Source: CAD feature listing. Evaluate the final solid. Frame: model axes, mm. Coordinates: 2 decimals unless noted, no trailing zeros. Write each loop counter-clockwise with the first axis right and the second up, starting at its lowest first coordinate (ties: lowest second). Pieces come first, ordered by that corner, then holes. Notation, with made-up numbers: (-7, 13) - (8, 13) arc R11 cw to (8, 17) - close; hole circle Ø10 at (44, 81.25). An arc over 180 degrees is marked (long way). One line per item, written item: value.
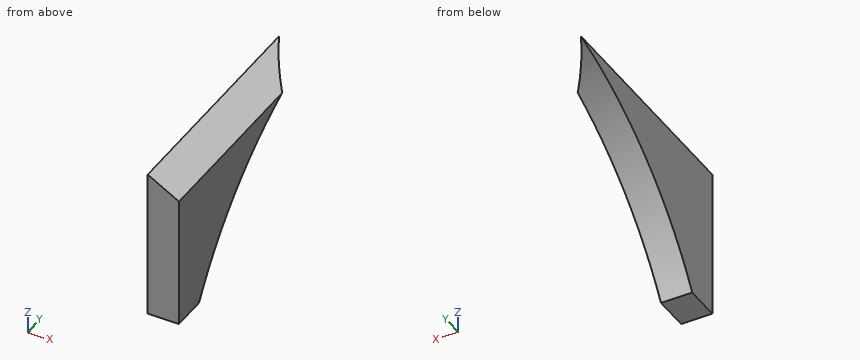
from build123d import *

# Parameters (mm, degrees)
BOSS_EXTRUDE1_DEPTH = 4
SKETCH2_W           = 10.75
SKETCH2_H           = 20.327264221
CUT_EXTRUDE1_DEPTH  = 4
CUT_EXTRUDE2_DEPTH  = 50.8


with BuildPart() as part:
    # Sketch1 → Boss-Extrude1 (new body)
    with BuildSketch(Plane(origin=(0, 0, 0), x_dir=(0, 0, -1), z_dir=(1, 0, 0))):
        with BuildLine():
            Line((-11.867139326, 22.331980986), (-11.867139326, -7.668019014))
            Line((-11.867139326, -7.668019014), (18.132860674, -7.668019014))
            ThreePointArc((18.132860674, -7.668019014), (-0.870157122, 3.328963189), (-11.867139326, 22.331980986))
        make_face()
    extrude(amount=BOSS_EXTRUDE1_DEPTH)

    # Sketch2 → Cut-Extrude1 (cut)
    with BuildSketch(Plane(origin=(4, 0, 0), x_dir=(0, 0, -1), z_dir=(1, 0, 0))):
        with Locations((12.757860674, 2.495613097)):
            Rectangle(SKETCH2_W, SKETCH2_H)
    extrude(amount=-CUT_EXTRUDE1_DEPTH, mode=Mode.SUBTRACT)

    # Sketch3 → Cut-Extrude2 (cut)
    with BuildSketch(Plane.XZ.offset(7.668019014)):
        Polygon((0, 11.867139326), (4, 9.557738249), (4, 11.867139326), align=None)
    extrude(amount=-CUT_EXTRUDE2_DEPTH, mode=Mode.SUBTRACT)


solid = part.part
1) Section query C-C on y = 18. Output: boundary loops of the cut face in (x, z).
Values found:
outline: (0, 10.44) - (2.46, 10.44) - (0, 11.87) - close
2) Material intervals for line 1 (Y direction, x = 0.55, z = -2.75); line 2 (Z direction, x = 1.15, y = -5.5); line 3 (Y direction, x = 3.7, z = -4), sorted ascending.
Values found:
line 1: -7.67 to 0.1
line 2: -7.38 to 11.2
line 3: -7.67 to -0.86
3) Section query B-B on x = 3.7. Output: boundary loops of the cut face in (y, z).
Values found:
outline: (-7.67, -7.38) - (-3.11, -7.38) arc R42.58 cw to (16.28, 9.73) - (-7.67, 9.73) - close
4) Section query A-A on y = -5.25. Output: boundary loops of the cut face in (x, z), then the cut area to 3 significant figures.
Values found:
outline: (0, -7.38) - (4, -7.38) - (4, 9.56) - (0, 11.87) - close
area: 72.4 mm2
5) Contact query for flat-ended pins moving along their axis: P1, Ø2, axis at x = 2, y = 11, coming from the +Z side; P2, Ø2, axis at x = 2, z = 3, coming from the +Y side; P3, Ø2, axis at x = 1, z = -5, coming from the +Y side. Output: stop coordinate, or through.
Values found:
P1: z = 11.29
P2: y = 6.82
P3: y = -0.86
